from build123d import *

# Parameters (mm, degrees)
F0_W     = 134.9375
F0_H     = 39.6875
F1_DEPTH = 74.6125
F2_W     = 128.5875
F2_H     = 68.2625
F3_DEPTH = 36.5125
F4_R     = 1.5875
F4_W     = 26.9875
F4_H     = 19.05
F5_DEPTH = 6.35
F6_R     = 6.35
F7_DEPTH = 6.35


with BuildPart() as f1:
    # F0 (on Front) → F1 (new body)
    with BuildSketch(Plane.XZ):
        with Locations((67.46875, 19.84375)):
            Rectangle(F0_W, F0_H)
    extrude(amount=-F1_DEPTH)

    # F2 (on face) → F3 (cut)
    with BuildSketch(Plane.XY.offset(39.6875)):
        with Locations((67.46875, 37.30625)):
            Rectangle(F2_W, F2_H)
    extrude(amount=-F3_DEPTH, mode=Mode.SUBTRACT)

    # F4 (on face) → F5 (cut)
    with BuildSketch(Plane.XZ):
        with Locations((12.7, 15.323338)):
            Circle(F4_R)
        with Locations((52.705, 15.323338)):
            Circle(F4_R)
        with Locations((32.18815, 15.323338)):
            Rectangle(F4_W, F4_H)
    extrude(amount=-F5_DEPTH, mode=Mode.SUBTRACT)

    # F6 (on face) → F7 (cut)
    with BuildSketch(Plane.XZ):
        with Locations((81.28, 15.3162)):
            Circle(F6_R)
    extrude(amount=-F7_DEPTH, mode=Mode.SUBTRACT)


solid = f1.part
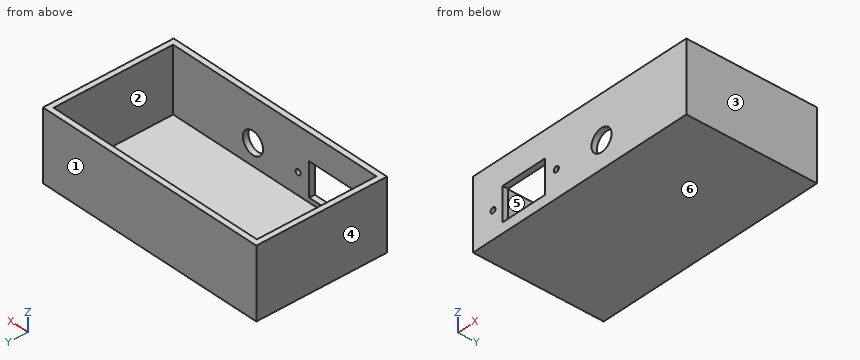
CAD build for the part. Positions are in the model's coordinates, mm. Face numbers are marked on the shaded views. A direction names the side the tool comes from. Round coordinates to 2 decimals unless told otherwise and drop trailing zeros. Write each loop counter-clockwise with the first axis right and the second up, starting at its lowest first coordinate (ties: lowest second). Pieces come first, ordered by that corner, then holes.
(1) Probe line 1 along X through (y, z) = (18.5, 19.5) (1 decimal); line 2 along Y through (x, z) = (105, 13) (1 decimal); line 3 along Z through (x, y) = (12.7, 1.45). List the from-to ranges inside material, lowest first.
(2) Slice it at D-D, the plane x = 48. Write the cut outline in (y, z) (1 decimal), and give its area (3 significant figures).
(3) Slice it at A-A, the plane x = 31.5. Write the cut outline in (y, z) (1 decimal).
(4) Mould opens along X. For the marked faces 3, 4, 5 and 6 say: pulls with the +X half, pulls with the -X half, needs draft (parallel to the pull), parting line crosses it, or undercut.
(5) Drop a flat-ended pin along its axis: P1, Ø20.5, axis at x = 82, y = 54, coming from the +Z side (3 decimals). Give the stop position or say it passes through.
(6) Slice it at C-C, the plane y = 39. Write the cut outline in (x, z) (1 decimal), and give its area (3 significant figures).
(7) 3-axis set-ups, long thin cutter, end or side, ignore diameter. For the marked faces 1 and 2: which of +Z, -Z, +X, -X, +Y, -Y reach the whole face in a straight line?
(8) Slice it at B-B, the plane z = 37. Write the cut outline in (x, y) (1 decimal).
From the geometry:
1. line 1: x = 0 to 3.2, 131.8 to 134.9
1. line 2: y = 0 to 3.2, 71.4 to 74.6
1. line 3: z = 0 to 13.74, 16.91 to 39.69
2. outline: (0, 0) - (74.6, 0) - (74.6, 39.7) - (71.4, 39.7) - (71.4, 3.2) - (3.2, 3.2) - (3.2, 39.7) - (0, 39.7) - close
2. area: 469 mm2
3. outline: (0, 0) - (74.6, 0) - (74.6, 39.7) - (71.4, 39.7) - (71.4, 3.2) - (3.2, 3.2) - (3.2, 5.8) - (0, 5.8) - close; (0, 24.8) - (3.2, 24.8) - (3.2, 39.7) - (0, 39.7) - close
4. face 3: pulls with the +X half
4. face 4: pulls with the -X half
4. face 5: undercut
4. face 6: needs draft
5. P1: stops at z = 3.175
6. outline: (0, 0) - (134.9, 0) - (134.9, 39.7) - (131.8, 39.7) - (131.8, 3.2) - (3.2, 3.2) - (3.2, 39.7) - (0, 39.7) - close
6. area: 660 mm2
7. face 1: +Z, -Z, +X, -X, +Y
7. face 2: +Z
8. outline: (0, 0) - (134.9, 0) - (134.9, 74.6) - (0, 74.6) - close; hole (3.2, 3.2) - (131.8, 3.2) - (131.8, 71.4) - (3.2, 71.4) - close
